Autodesk Fusion 360 part; units mm, degrees
sketch "Sketch1" plane through (0, 0, 0) normal (0, 0, 1) x (1, 0, 0)
  line L0 (-84.8651, 33.3057) -> (-69.0651, 33.3057)
  line L1 (-69.0651, 33.3057) -> (-69.0651, 17.5057)
  line L2 (-69.0651, 17.5057) -> (-84.8651, 17.5057)
  line L3 (-84.8651, 17.5057) -> (-84.8651, 33.3057)
  line L4 (-84.8651, 33.3057) -> (-69.0651, 17.5057) construction
  line L5 (-69.0651, 33.3057) -> (-84.8651, 17.5057) construction
  line L6 (-50.0651, 33.3057) -> (-50.0651, 17.5057)
  line L7 (-65.8651, 33.3057) -> (-50.0651, 33.3057)
  line L8 (-65.8651, 17.5057) -> (-65.8651, 33.3057)
  line L9 (-50.0651, 17.5057) -> (-65.8651, 17.5057)
  line L10 (-31.0651, 33.3057) -> (-31.0651, 17.5057)
  line L11 (-46.8651, 33.3057) -> (-31.0651, 33.3057)
  line L12 (-46.8651, 17.5057) -> (-46.8651, 33.3057)
  line L13 (-31.0651, 17.5057) -> (-46.8651, 17.5057)
  line L14 (-12.0651, 33.3057) -> (-12.0651, 17.5057)
  line L15 (-27.8651, 33.3057) -> (-12.0651, 33.3057)
  line L16 (-27.8651, 17.5057) -> (-27.8651, 33.3057)
  line L17 (-12.0651, 17.5057) -> (-27.8651, 17.5057)
  line L18 (-69.0651, 52.3057) -> (-69.0651, 36.5057)
  line L19 (-84.8651, 52.3057) -> (-69.0651, 52.3057)
  line L20 (-84.8651, 36.5057) -> (-84.8651, 52.3057)
  line L21 (-69.0651, 36.5057) -> (-84.8651, 36.5057)
  line L22 (-50.0651, 52.3057) -> (-50.0651, 36.5057)
  line L23 (-65.8651, 52.3057) -> (-50.0651, 52.3057)
  line L24 (-65.8651, 36.5057) -> (-65.8651, 52.3057)
  line L25 (-50.0651, 36.5057) -> (-65.8651, 36.5057)
  line L26 (-31.0651, 52.3057) -> (-31.0651, 36.5057)
  line L27 (-46.8651, 52.3057) -> (-31.0651, 52.3057)
  line L28 (-46.8651, 36.5057) -> (-46.8651, 52.3057)
  line L29 (-31.0651, 36.5057) -> (-46.8651, 36.5057)
  line L30 (-12.0651, 52.3057) -> (-12.0651, 36.5057)
  line L31 (-27.8651, 52.3057) -> (-12.0651, 52.3057)
  line L32 (-27.8651, 36.5057) -> (-27.8651, 52.3057)
  line L33 (-12.0651, 36.5057) -> (-27.8651, 36.5057)
  line L34 (-86.8651, 54.3057) -> (-10.0651, 54.3057)
  line L35 (-10.0651, 54.3057) -> (-10.0651, 15.5057)
  line L36 (-10.0651, 15.5057) -> (-86.8651, 15.5057)
  line L37 (-86.8651, 15.5057) -> (-86.8651, 54.3057)
  point P0 (-76.9651, 25.4057)
  dimension "d3" = 15.8
  dimension "d4" = 15.8
  dimension "d7" = 19
  dimension "d8" = 19
  dimension "d9" = 2
  dimension "d10" = 2
  dimension "d11" = 2
  dimension "d12" = 2
extrude "Extrude1" add sketch "Sketch1" along normal blind 10
Check sheet for the modelled part. Datum: model origin and axes. Units: mm. A direction names the side the tool comes from. Coordinates: 2 decimals unless noted, no trailing zeros. Write each loop counter-clockwise with the first axis right and the second up, starting at its lowest first coordinate (ties: lowest second). Pieces come first, ordered by that corner, then holes. Notation, with made-up numbers: M 76.5,5.5 L 111.5,5.5 A23 ccw 111.5,35.5 Z; hole C 46,17.25 d2. An arc over 180 degrees is marked long. Write item = value, one per line. Start each with the question number.
1. Thickness scan on probe 1 along Y at (x, z) = (-17.5, 7.5); probe 2 along X at (y, z) = (28, 7.75). Record the ranges inside material, lowest first.
2. Sectioned sample at C-C (z = 6.25). State how many separate pieces and enclosed holes the cut face has, then the cut area to 3 significant figures.
3. Sectioned sample at A-A (y = 38). Record the cut outline in (x, z), then the cut area to 3 significant figures.
4. Sectioned sample at B-B (x = -80). Record the cut outline in (y, z), then the cut area to 3 significant figures.
5. Tool access check on faces 1 (the flat face through (-48, 15.506, 5)), 2 (the flat face through (-39, 17.506, 5)). Record the directions out of +Z, -Z, +X, -X, +Y, -Y that give a thin tool (end or side, any length) a straight path to the whole face; none if there is none.
The answers:
q1.probe_1 = 15.51 to 17.51, 33.31 to 36.51, 52.31 to 54.31
q1.probe_2 = -86.87 to -84.87, -69.07 to -65.87, -50.07 to -46.87, -31.07 to -27.87, -12.07 to -10.07
q2.separate_pieces = 1
q2.enclosed_holes = 8
q2.area = 983 mm²
q3.outline = M -86.87,0 L -84.87,0 L -84.87,10 L -86.87,10 Z; M -69.07,0 L -65.87,0 L -65.87,10 L -69.07,10 Z; M -50.07,0 L -46.87,0 L -46.87,10 L -50.07,10 Z; M -31.07,0 L -27.87,0 L -27.87,10 L -31.07,10 Z; M -12.07,0 L -10.07,0 L -10.07,10 L -12.07,10 Z
q3.area = 136 mm²
q4.outline = M 15.51,0 L 17.51,0 L 17.51,10 L 15.51,10 Z; M 33.31,0 L 36.51,0 L 36.51,10 L 33.31,10 Z; M 52.31,0 L 54.31,0 L 54.31,10 L 52.31,10 Z
q4.area = 72.0 mm²
q5.face_1 = +Z, -Z, +X, -X, -Y
q5.face_2 = +Z, -Z
